```python
from build123d import *

# Parameters (mm, degrees)
BOSS_EXTRUDE1_DEPTH = 3
BOSS_EXTRUDE2_DEPTH = 12
SKETCH8_R           = 2
CUT_EXTRUDE2_DEPTH  = 27.616080544


with BuildPart() as part:
    # Sketch1 → Boss-Extrude1 (new body)
    with BuildSketch(Plane.XY):
        Polygon((15.219519397, 37.989351506), (20.219519397, 37.989351506), (20.219519397, 32.909351506), (15.219519397, 32.909351506), (15.219519397, 25.341157087), (20.219519397, 25.341157087), (20.219519397, 20.261157087), (15.219519397, 20.261157087), (15.219519397, 16.399351506), (0, 10.609645279), (-2.165979283, 49.840454802), align=None)
    extrude(amount=BOSS_EXTRUDE1_DEPTH)

    # Sketch7 → Boss-Extrude2 (add)
    with BuildSketch(Plane(origin=(0, 0, 0), x_dir=(-1, 0, 0), z_dir=(0, 0, -1))):
        Polygon((-7.622037061, 31.367483037), (-6.766619255, 34.559945753), (-0.453977977, 32.868478621), (-1.309395784, 29.676015905), align=None)
        Polygon((-8.709077051, 27.310594567), (-2.396435773, 25.619127434), (-3.25185358, 22.426664718), (-9.564494858, 24.118131851), align=None)
    extrude(amount=BOSS_EXTRUDE2_DEPTH)

    # Sketch8 → Cut-Extrude2 (cut, through all)
    with BuildSketch(Plane(origin=(-8.186708897, 30.553213551, 0), x_dir=(0.965925826, 0.258819045, 0), z_dir=(-0.258819045, 0.965925826, 0))):
        with Locations((12.213160878, 8.044397723)):
            Circle(SKETCH8_R)
    extrude(amount=-CUT_EXTRUDE2_DEPTH, mode=Mode.SUBTRACT)


solid = part.part
```
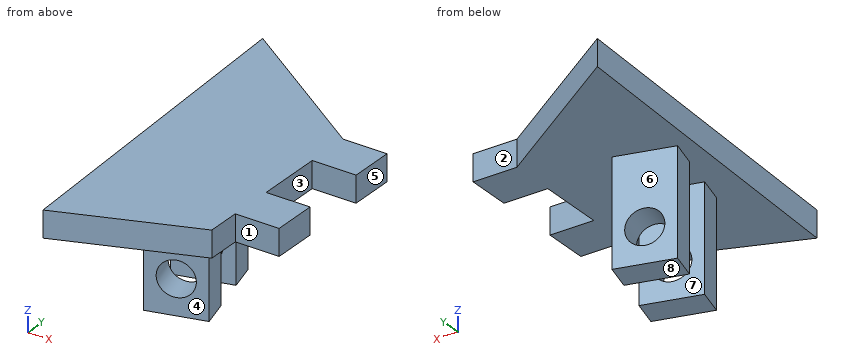
The listing builds one solid part. Answer for the finished solid, in the listing's coordinates (mm). Face numbers are marked on the shaded views. A direction names the side the tool comes from. Coordinates: 2 decimals unless noted, no trailing zeros. Loops run counter-clockwise (first coordinate to the right, second up) from the corner with the lowest first, then second, coordinate; pieces in that order, holes last. Notation, with made-up numbers: M 5,40.5 L 54,40.5 A18 ccw 54,70.5 Z; hole C 51,70 d11. An arc over 180 degrees is marked long. Answer as CSV lines item,"result". Start each with the question number.
(1) For the marked faces 1, 2, 3, 4 and 5, determine the directions among +Z, -Z, +X, -X, +Y, -Y from which every point of the face is accessible in a straight line to the end or side of a thin tool.
(2) The part is cut by section B-B (z = 0.75). Give the vertices of the cut face in (x, y).
(3) The part is cut by section C-C (x = 5). State how many separate pieces and enclosed holes the cut face has, and give its area (3 significant figures).
(4) Given pin 1 (2.5 mm diameter, centred on x = 16.5, z = 1, fed in from -Y); pin 2 (1.5 mm diameter, centred on y = 28, z = 1, fed in from +X); pin 3 (0.9 mm diameter, centred on x = 18.5, z = 1.5, fed in from +Y), each flat-ended and moving along its own axis, determine where each tip first touches the part or whether it passes through.
(5) The part is cut by section D-D (y = 44). Give the vertices of the cut face in (x, z).
(6) The part is cut by section A-A (x = 17). Give the vertices of the cut face in (y, z), and give its area (3 significant figures).
(7) The mould has two halves that part along Y. Classify the marked faces 6, 7 and 8: pulls with the +Y half, pulls with the -Y half, needs draft (parallel to the pull), parting line crosses it, or undercut.
(8) Find the intervals of material crossed by L1, parallel to Z at x = 3.25, y = 27.5; L2, parallel to X at y = 35.5, z = 0.75; L3, parallel to X at y = 25, z = 2, in increasing order. Write a range as [from, to].
Determined:
1,face 1,"+Z, -Z, +X, -Y"
1,face 2,"+Z, -Z, +X, +Y"
1,face 3,"+Z, -Z, +X"
1,face 4,"-Z, +X, -Y"
1,face 5,"+Z, -Z, +X, +Y, -Y"
2,outline,"M -2.17,49.84 L 0,10.61 L 15.22,16.4 L 15.22,20.26 L 20.22,20.26 L 20.22,25.34 L 15.22,25.34 L 15.22,32.91 L 20.22,32.91 L 20.22,37.99 L 15.22,37.99 Z"
3,separate pieces,"3"
3,enclosed holes,"0"
3,area,"156 mm2"
4,pin 1,"y = 20.26"
4,pin 2,"x = 15.22"
4,pin 3,"y = 37.99"
5,outline,"M -1.84,0 L 6.4,0 L 6.4,3 L -1.84,3 Z"
6,outline,"M 20.26,0 L 25.34,0 L 25.34,3 L 20.26,3 Z; M 32.91,0 L 37.99,0 L 37.99,3 L 32.91,3 Z"
6,area,"30.5 mm2"
7,face 6,"pulls with the +Y half"
7,face 7,"undercut"
7,face 8,"needs draft"
8,L1,"[0, 3]"
8,L2,"[-1.37, 20.22]"
8,L3,"[-0.79, 20.22]"
